Autodesk Fusion 360 part; units mm, degrees
sketch "Sketch1" plane through (0, 0, 0) normal (0, 0, 1) x (1, 0, 0)
  line L0 (-40, -30) -> (-40, 22.5)
  line L1 (-9.9671, 30) -> (10, 30)
  line L2 (40, 22.5) -> (40, -30)
  line L3 (25, -30) -> (25, -4.623)
  line L4 (-25, -4.623) -> (-25, -30)
  line L5 (40, -30) -> (25, -30)
  line L6 (-25, -30) -> (-40, -30)
  line L7 (10, -4.623) -> (10, 15)
  line L8 (10, 15) -> (-9.9671, 15)
  line L9 (-9.9671, 15) -> (-9.9671, -4.623)
  line L10 (10, 22.5) -> (10, 30)
  line L11 (-9.9671, 22.5) -> (-9.9671, 30)
  line L12 (10, 22.5) -> (40, 22.5)
  line L13 (-9.9671, 22.5) -> (-40, 22.5)
  line L14 (25, -4.623) -> (10, -4.623)
  line L15 (-9.9671, -4.623) -> (-25, -4.623)
extrude "Extrude1" add sketch "Sketch1" along normal mid plane 170
sketch "Sketch2" plane through (0, 0, 85) normal (0, 0, 1) x (1, 0, 0)
  line L0 (10, 22.5) -> (10, 30)
  line L1 (10, 30) -> (-9.9671, 30)
  line L2 (-9.9671, 30) -> (-9.9671, 22.5)
  line L3 (-9.9671, 22.5) -> (-40, 22.5)
  line L4 (-40, 22.5) -> (-40, -30)
  line L5 (-40, -30) -> (-25, -30)
  line L6 (-25, -30) -> (-25, -4.623)
  line L7 (-25, -4.623) -> (-9.9671, -4.623)
  line L8 (-9.9671, -4.623) -> (-9.9671, 15)
  line L9 (-9.9671, 15) -> (10, 15)
  line L10 (10, 15) -> (10, -4.623)
  line L11 (10, -4.623) -> (25, -4.623)
  line L12 (25, -4.623) -> (25, -30)
  line L13 (25, -30) -> (40, -30)
  line L14 (40, -30) -> (40, 22.5)
  line L15 (40, 22.5) -> (10, 22.5)
  line L16 (-40, 22.5) -> (-40, 35)
  line L17 (-40, 35) -> (40, 35)
  line L18 (40, 35) -> (40, 22.5)
extrude "Extrude2" add sketch "Sketch2" against normal blind 40 contours L0 L1 L2 L3 L15 L16 L17 L18
sketch "Sketch3" plane through (40, 0, 0) normal (1, 0, 0) x (0, 0, -1)
  line L0 (85, 22.5) -> (-45, 22.5)
  line L1 (-45, 22.5) -> (-45, 35)
  line L2 (-45, 35) -> (-85, 35)
  line L3 (-85, 35) -> (-85, -30)
  line L4 (-85, -30) -> (85, -30)
  line L5 (85, -30) -> (85, 22.5)
  line L6 (-45, 35) -> (-45, 70)
  arc A0 (-45, 70) -> (-80, 35) centre (-45, 35) ccw
extrude "Extrude3" add sketch "Sketch3" against normal up to surface (80 mm away) contours L2 L6 A0
sketch "Sketch4" plane through (0, 0, -85) normal (0, 0, -1) x (-1, 0, 0)
  line L0 (-10, 30) -> (-10, 22.5)
  line L1 (-10, 22.5) -> (-40, 22.5)
  line L2 (-40, 22.5) -> (-40, -30)
  line L3 (-40, -30) -> (-25, -30)
  line L4 (-25, -30) -> (-25, -4.623)
  line L5 (-25, -4.623) -> (-10, -4.623)
  line L6 (-10, -4.623) -> (-10, 15)
  line L7 (-10, 15) -> (9.9671, 15)
  line L8 (9.9671, 15) -> (9.9671, -4.623)
  line L9 (9.9671, -4.623) -> (25, -4.623)
  line L10 (25, -4.623) -> (25, -30)
  line L11 (25, -30) -> (40, -30)
  line L12 (40, -30) -> (40, 22.5)
  line L13 (40, 22.5) -> (9.9671, 22.5)
  line L14 (9.9671, 22.5) -> (9.9671, 30)
  line L15 (9.9671, 30) -> (-10, 30)
  line L16 (-40, 22.5) -> (-40, 45)
  line L17 (40, 45) -> (40, 22.5)
  arc A0 (25, 45) -> (-25, 45) centre (0, 45) ccw
  line L18 (-40, 45) -> (-25, 45)
  line L19 (25, 45) -> (40, 45)
extrude "Extrude4" add sketch "Sketch4" against normal blind 35 contours L0 L1 L13 L14 L15 L16 L17 A0 L18 L19
Read the model definition and answer for the solid it produces. Units are mm, in the model's axes. A direction names the side the tool comes from. Give positions to 0.01 mm unless a question says otherwise; leave off trailing zeros. Write each loop counter-clockwise with the first axis right and the second up, starting at its lowest first coordinate (ties: lowest second). Pieces come first, ordered by that corner, then holes. Notation, with made-up numbers: M 85.25,80 L 136.25,80 A20 cw 136.25,119 Z; hole C 28,-9.75 d7. An arc over 180 degrees is marked long. Put each result on its own line as item: value. Start each with the question number.
1. The part is cut by section A-A, the plane y = 1.5. Give the vertices of the cut face in (x, z).
2. Consider line 1 along Z through (x, y) = (14.5, 28.5); line 2 along X through (y, z) = (-3.5, -70); line 3 along X through (y, z) = (-19, 37.5). Determine where each line is inside the solid, lowest interval first.
3. Each of these flat-tipped pins is pushed along its axis until it touches: pin 1 Ø1.5 at (x, z) = (27, 43) entering from +Y; pin 2 Ø22 at (x, z) = (3.5, 36.5) entering from -Y; pin 3 Ø6 at (x, z) = (-4.5, -25.5) entering from +Y. Where does it stop, or does it pass through?
4. The part is cut by section D-D, the plane x = -27.5. Give the vertices of the cut face in (y, z).
5. The part is cut by section C-C, the plane z = 11.5. Give the vertices of the cut face in (x, y), and give its area (3 significant figures).
6. The part is cut by section B-B, the plane x = 0. Give the vertices of the cut face in (y, z), and give its area (3 significant figures).
7. Which of the six approach directions +Z, -Z, +X, -X, +Y, -Y give full straight-line access (tool end or side, diameter ignored) to faces 1 (the flat face through (-32, 45, -68)), 2 (the flat face through (18, -4.623, -1)), 3 (the flat face through (25, 22.5, -3))?
8. For a pull along X with two mould halves and no side action, classify faces 4 (the flat face through (1, 46, 45)), 5 (the flat face through (-25, -17, -1)), 6 (the cylindrical face through (-0.55, 69.994, -67.745)) as released by +X, released by -X, zero draft, split by the parting line, or undercut.
Final values:
1. outline: M -40,-85 L -9.97,-85 L -9.97,85 L -40,85 Z; M 10,-85 L 40,-85 L 40,85 L 10,85 Z
2. line 1: z = -85 to -50, 45 to 85
2. line 2: x = -40 to -9.97, 10 to 40
2. line 3: x = -40 to -25, 25 to 40
3. pin 1: stops at y = 22.5
3. pin 2: stops at y = -4.62
3. pin 3: stops at y = 30
4. outline: M -30,-85 L 45,-85 L 45,-50 L 22.5,-50 L 22.5,45 L 70,45 A35 ccw 35,80 L 35,85 L -30,85 Z
5. outline: M -40,-30 L -25,-30 L -25,-4.62 L -9.97,-4.62 L -9.97,15 L 10,15 L 10,-4.62 L 25,-4.62 L 25,-30 L 40,-30 L 40,22.5 L 10,22.5 L 10,30 L -9.97,30 L -9.97,22.5 L -40,22.5 Z
5. area: 2,690 mm²
6. outline: M 15,-85 L 70,-85 L 70,-50 L 30,-50 L 30,45 L 70,45 A35 ccw 35,80 L 35,85 L 15,85 Z
6. area: 5,110 mm²
7. face 1: -Z, -X, +Y
7. face 2: +Z, -Z, -Y
7. face 3: +X, +Y
8. face 4: zero draft
8. face 5: undercut
8. face 6: split by the parting line
